Could you check a few things on this model? Use its own coordinates, in mm. Face numbers are marked on the shaded views. Coordinates: 2 decimals unless noted, no trailing zeros. Write each loop counter-clockwise with the first axis right and the second up, starting at its lowest first coordinate (ties: lowest second). Pieces come first, ordered by that corner, then holes. Notation, with made-up numbers: M 4,-1 L 20,-1 A19 cw 20,24 Z; hole C -33,-30.5 d7. An arc over 180 degrees is marked long. Write item = value, one per line.
```python
from build123d import *

# Parameters (mm, degrees)
F0_W      = 139.192
F0_H      = 69.342
F1_DEPTH  = 13.716
F2_W      = 123.698
F2_H      = 58.674
F3_DEPTH  = 7.62
F4_R      = 12.7
F5_R      = 12.7
F6_W      = 40.32391496
F6_H      = 5.8811781928
F7_DEPTH  = 25.4
F8_W      = 32.8259784728
F8_H      = 7.62
F9_DEPTH  = 25.4
F10_W     = 5.334
F10_H     = 1.2496084515
F11_DEPTH = 33.02
F12_W     = 9.6497610211
F12_H     = 18.7207064591
F13_DEPTH = 25.4
F14_R     = 2.54
F15_W     = 11.7547400296
F15_H     = 4.3837525882
F16_DEPTH = 25.4
F17_R     = 1.27
F18_SIZE  = 5.08
F19_DEPTH = 2.54
F20_R     = 5.08
F21_DEPTH = 1.778
F22_DEPTH = 1.778


with BuildPart() as f1:
    # F0 (on Top) → F1 (new body)
    with BuildSketch(Plane.XY):
        Rectangle(F0_W, F0_H)
    extrude(amount=F1_DEPTH)

    # F2 (on face) → F3 (cut)
    with BuildSketch(Plane.XY.offset(13.716)):
        Rectangle(F2_W, F2_H)
    extrude(amount=-F3_DEPTH, mode=Mode.SUBTRACT)

    # F4
    f4_edges = [f1.edges().sort_by_distance(p)[0] for p in [
        (69.596, -34.671, 6.858),
    ]]
    fillet(f4_edges, radius=F4_R)

    # F5
    f5_edges = [f1.edges().sort_by_distance(p)[0] for p in [
        (69.596, 34.671, 6.858),
        (-69.596, -34.671, 6.858),
        (-69.596, 34.671, 6.858),
    ]]
    fillet(f5_edges, radius=F5_R)

    # F6 (on face) → F7 (cut)
    with BuildSketch(Plane.YZ.offset(69.596)):
        with Locations((-0.1104911789, 9.7644287162)):
            Rectangle(F6_W, F6_H)
    extrude(amount=-F7_DEPTH, mode=Mode.SUBTRACT)

    # F8 (on face) → F9 (cut)
    with BuildSketch(Plane(origin=(0, -29.337, 0), x_dir=(-1, 0, 0), z_dir=(0, 1, 0))):
        with Locations((38.5076953098, 9.906)):
            Rectangle(F8_W, F8_H)
    extrude(amount=-F9_DEPTH, mode=Mode.SUBTRACT)

    # F10 (on face) → F11 (join)
    with BuildSketch(Plane.YZ.offset(-54.9206845462)):
        with Locations((-32.004, 13.0911957743)):
            Rectangle(F10_W, F10_H)
    extrude(amount=F11_DEPTH)

    # F12 (on face) → F13 (cut)
    with BuildSketch(Plane(origin=(0, 0, 0), x_dir=(1, 0, 0), z_dir=(0, 0, -1))):
        with Locations((-56.7813999951, -16.70263079)):
            Rectangle(F12_W, F12_H)
    extrude(amount=-F13_DEPTH, mode=Mode.SUBTRACT)

    # F14
    f14_edges = [f1.edges().sort_by_distance(p)[0] for p in [
        (-51.956519, 7.342278, 3.048),
        (-61.606281, 26.062984, 3.048),
        (-61.606281, 7.342278, 3.048),
        (-51.956519, 26.062984, 3.048),
    ]]
    fillet(f14_edges, radius=F14_R)

    # F15 (on face) → F16 (cut)
    with BuildSketch(Plane.YZ.offset(-61.849)):
        with Locations((18.2274878025, 9.8191385623)):
            Rectangle(F15_W, F15_H)
    extrude(amount=-F16_DEPTH, mode=Mode.SUBTRACT)

    # F17
    f17_edges = [f1.edges().sort_by_distance(p)[0] for p in [
        (-65.7225, 12.350118, 7.627262),
        (-65.7225, 12.350118, 12.011015),
        (-65.632225, 24.104858, 7.627262),
        (-65.632225, 24.104858, 12.011015),
    ]]
    fillet(f17_edges, radius=F17_R)

    # F18
    f18_edges = [f1.edges().sort_by_distance(p)[0] for p in [
        (0, -34.671, 0),
    ]]
    chamfer(f18_edges, length=F18_SIZE)

    # F19 (cut): a face of the model
    f19_faces = [f1.faces().sort_by_distance(p)[0] for p in [
        (-61.849, -2.3026136032, 9.916972896),
    ]]
    extrude(f19_faces, amount=-F19_DEPTH, mode=Mode.SUBTRACT)

    # F20
    f20_edges = [f1.edges().sort_by_distance(p)[0] for p in [
        (-64.389, -29.337, 9.906),
        (-64.389, 29.337, 9.906),
        (61.849, -29.337, 9.906),
        (61.849, 29.337, 9.906),
    ]]
    fillet(f20_edges, radius=F20_R)

    # F21 (add): a face of the model
    f21_faces = [f1.faces().sort_by_distance(p)[0] for p in [
        (-54.9206845462, -32.004, 9.2811957743),
    ]]
    extrude(f21_faces, amount=F21_DEPTH)

    # F22 (cut): a face of the model
    f22_faces = [f1.faces().sort_by_distance(p)[0] for p in [
        (-22.0947060734, -32.004, 9.2811957743),
    ]]
    extrude(f22_faces, amount=-F22_DEPTH, mode=Mode.SUBTRACT)


solid = f1.part
```
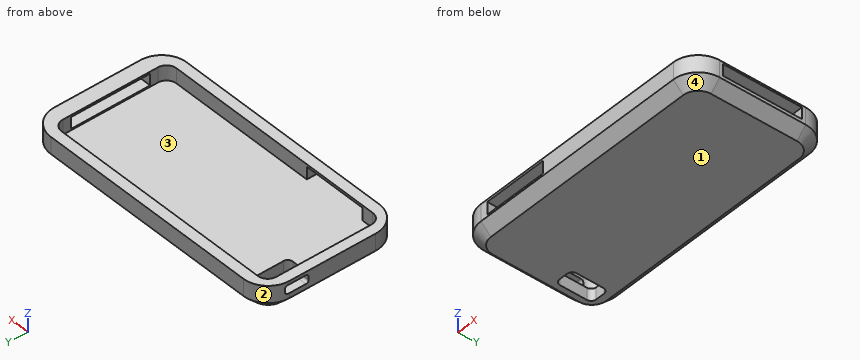
Item 1: I'm going to push flat-ended pins straight in: P1, Ø6.5, axis at y = 14, z = 2.5, coming from the +X side; P2, Ø1.4, axis at x = -56, z = 3.5, coming from the -Y side; P3, Ø1.8, axis at x = 66.5, z = 9, coming from the -Y side; P4, Ø19, axis at x = -13, y = -17, coming from the +Z side. Where does each tip first touch, or does it pass through?
Numbers:
P1 = 69.6
P2 = -33.79
P3 = -31.22
P4 = 6.1
Item 2: Imagine slicing it at A-A (y = -5). Write out the boundary of the cut face in (x, z).
Numbers:
outline = M -69.6,5.08 L -64.52,0 L 64.52,0 L 69.6,5.08 L 69.6,6.82 L 61.85,6.82 L 61.85,6.1 L -64.39,6.1 L -64.39,13.72 L -69.6,13.72 Z; M 61.85,12.71 L 69.6,12.71 L 69.6,13.72 L 61.85,13.72 Z
Item 3: If we mould it in two halves opening along X, with no side actions, what happens to the marked faces 1, 2, 3 and 4? For each: pulls with the +X half, pulls with the -X half, needs draft (parallel to the pull), parting line crosses it, or undercut.
Numbers:
face_1 = needs draft
face_2 = pulls with the -X half
face_3 = undercut
face_4 = pulls with the +X half
Item 4: Imagine slicing it at B-B (z = 2). Write out the boundary of the cut face in (x, y).
Numbers:
outline = M -66.52,-21.97 A9.62 ccw -56.9,-31.59 L 56.9,-31.59 A9.62 ccw 66.52,-21.97 L 66.52,21.97 A9.62 ccw 56.9,31.59 L -56.9,31.59 A9.62 ccw -66.52,21.97 Z; hole M -61.61,9.88 A2.54 ccw -59.07,7.34 L -54.5,7.34 A2.54 ccw -51.96,9.88 L -51.96,23.52 A2.54 ccw -54.5,26.06 L -59.07,26.06 A2.54 ccw -61.61,23.52 Z
Item 5: Imagine slicing it at C-C (x = 17). Write out the boundary of the cut face in (y, z).
Numbers:
outline = M -34.67,5.08 L -29.59,0 L 29.59,0 L 34.67,5.08 L 34.67,13.72 L 29.34,13.72 L 29.34,6.1 L -29.34,6.1 L -29.34,13.72 L -34.67,13.72 Z
Item 6: If I drill on line 1 along Y through (x, z) = (-18, 12.5); line 2 along X through (y, z) = (-3, 6.75); line 3 along X through (y, z) = (14, 5.25), over which ranges is the centre line in solid material (lowest first)?
Numbers:
line_1 = -34.67 to -29.34, 29.34 to 34.67
line_2 = -69.6 to -64.39, 61.85 to 69.6
line_3 = -69.6 to -61.61, -51.96 to 69.6
